from build123d import *

# Parameters (mm, degrees)
F0_R     = 380.9365
F0_R_2   = 236.5375
F1_DEPTH = 304.8
F6_W     = 53.241849
F6_H     = 17.892758
F7_DEPTH = 231.14


with BuildPart() as f1:
    # F0 (on Front) → F1 (new body)
    with BuildSketch(Plane.XZ):
        Circle(F0_R)
        Circle(F0_R_2, mode=Mode.SUBTRACT)
    extrude(amount=-F1_DEPTH)

    # F2 (on Right) → F3 (revolve, cut)
    with BuildSketch(Plane.YZ):
        Polygon((-0.674657, 0), (0, 0), (9.525, 0), (9.525, 323.444068), (0, 325.9074), (-38.13795, 325.9074), align=None)
    revolve(axis=Axis((0, -111.905819, 0), (0, -1, 0)), mode=Mode.SUBTRACT)

    # F4 (on Right) → F5 (revolve, cut)
    with BuildSketch(Plane.YZ):
        Polygon((39.294728, 254.3556), (9.525, 266.9921), (-83.954796, 266.9921), (-48.076838, 187.997639), (83.789648, 229.984577), (72.7964, 240.977825), (52.705, 252.5776), (45.438306, 252.5776), (41.2496, 254.3556), align=None)
    revolve(axis=Axis((0, 0, 0), (0, -1, 0)), mode=Mode.SUBTRACT)

    # F6 (on Top) → F7 (cut)
    with BuildSketch(Plane.XY):
        with Locations((-368.849694, -4.439522)):
            Rectangle(F6_W, F6_H)
    extrude(amount=-F7_DEPTH, mode=Mode.SUBTRACT)


solid = f1.part
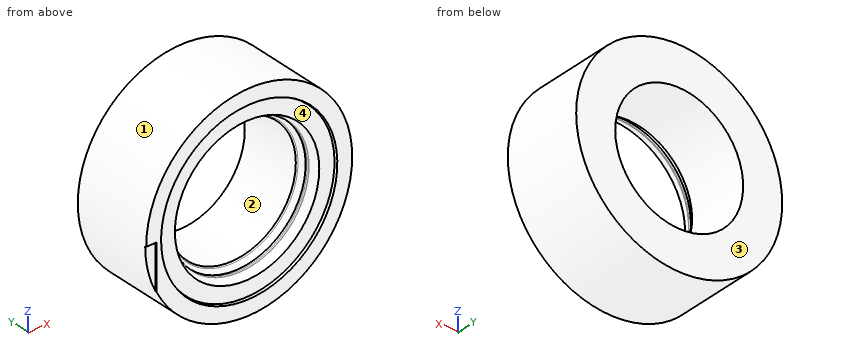
The model under review builds one solid part; all positions refer to its coordinate system, in mm. Face numbers are marked on the shaded views. Give positions to 0.01 mm unless a question says otherwise; leave off trailing zeros. Write each loop counter-clockwise with the first axis right and the second up, starting at its lowest first coordinate (ties: lowest second). Pieces come first, ordered by that corner, then holes.
1. Add section A-A, the plane x = 0. Write out the cut boundary in (y, z) (1 decimal), plus the area to 3 significant figures.
2. Add section B-B, the plane y = 94.5. Write out the cut boundary in (x, z) (1 decimal).
3. For P1, Ø12, axis at y = 243.5, z = -236.5, coming from the +X side; P2, Ø10, axis at y = 74.5, z = 196, coming from the -X side; P3, Ø1.5, axis at y = 202.5, z = -102.5, coming from the +X side, all flat-tipped, find the tip position at first contact; note any pin that passes through.
4. Draft analysis for pull direction Z (two halves, no side actions). For the marked faces 1, 2, 3 and 4, state which applies: +Z half, -Z half, draft (parallel to the pull), parting line (faces both ways), or undercut.
5. Wall thickness on L1, parallel to Z at x = 0, y = 245.5; L2, parallel to Z at x = 0, y = 50.5; L3, parallel to X at y = 39.7, z = 0: over which ranges is each line inside the solid? List them lowest first.
Worked answers:
1. outline: (0, -380.9) - (304.8, -380.9) - (304.8, -236.5) - (77.2, -236.5) - (72.8, -241) - (52.7, -252.6) - (45.4, -252.6) - (41.2, -254.4) - (39.3, -254.4) - (9.5, -267) - (9.5, -323.4) - (0, -325.9) - close; (0, 325.9) - (9.5, 323.4) - (9.5, 267) - (39.3, 254.4) - (41.2, 254.4) - (45.4, 252.6) - (52.7, 252.6) - (72.8, 241) - (77.2, 236.5) - (304.8, 236.5) - (304.8, 380.9) - (0, 380.9) - close
1. area: 84,000 mm2
2. outline: circle Ø761.9 at (0, 0); hole circle Ø473.1 at (0, 0)
3. P1: stops at x = 303.29
3. P2: stops at x = -329.59
3. P3: stops at x = 367.1
4. face 1: parting line
4. face 2: undercut
4. face 3: draft
4. face 4: undercut
5. L1: z = -380.94 to -236.54, 236.54 to 380.94
5. L2: z = -380.94 to -252.58, 252.58 to 380.94
5. L3: x = -380.94 to -254.36, 254.36 to 380.94
